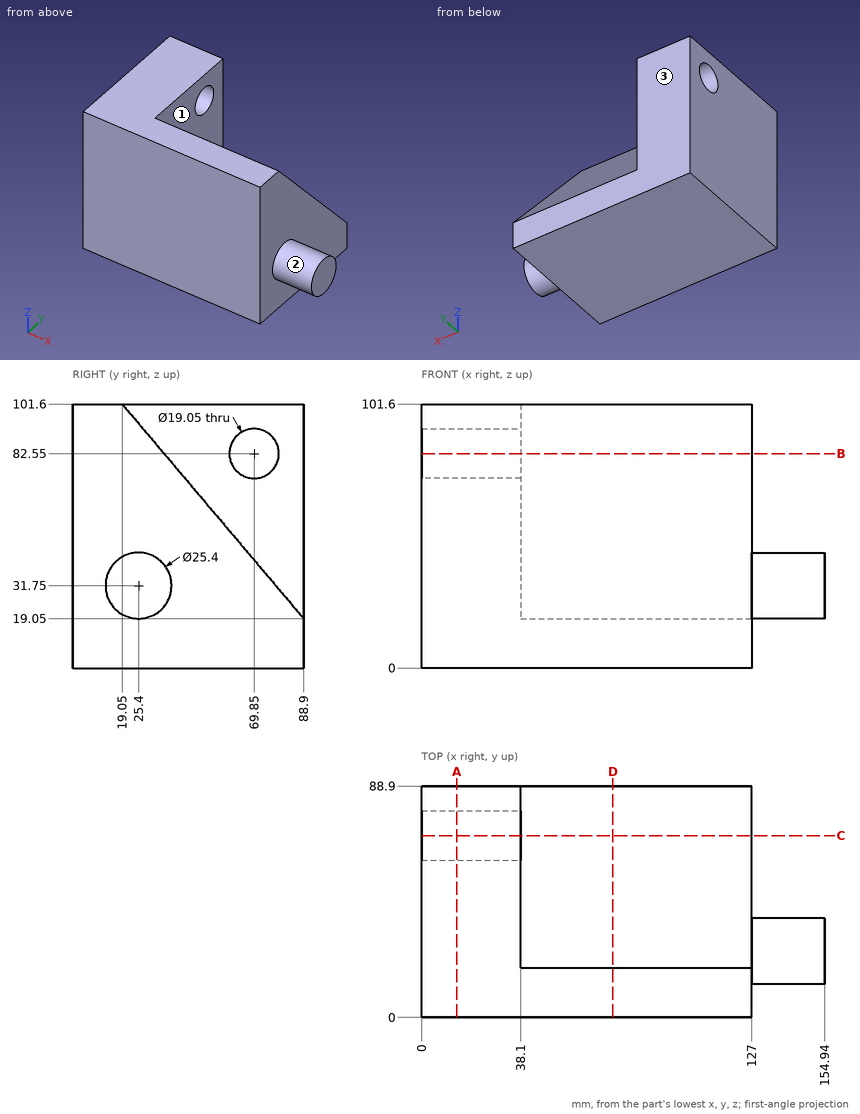
Answer from the drawing. Dimensions are ordinates in mm from the lowest x, y and z of the part. A direction names the side the tool comes from. Give positions to 0.01 mm unless a question says otherwise; leave off trailing zeros. Loops run counter-clockwise (first coordinate to the right, second up) from the corner with the lowest first, then second, coordinate; pieces in that order, holes last. Notation, with made-up numbers: M -28.5,61.25 L -1.5,61.25 A19 cw -1.5,73.25 Z; hole C -2.75,69 d6. An arc over 180 degrees is marked long. One line per item, written item: value.
Q1. A cutting plane is placed at D-D on x = 73.5. Determine the outline of the cut face in (y, z).
Working result:
outline: M 0,0 L 88.9,0 L 88.9,19.05 L 19.05,101.6 L 0,101.6 Z
Q2. Flat-ended cylindrical pins translate along their axes: P1, Ø1.5, axis at x = 108.5, y = 30.5, coming from the +Z side; P2, Ø21, axis at y = 56, z = 62, coming from the +X side; P3, Ø3, axis at x = 99, y = 75.5, coming from the +Z side; P4, Ø3, axis at y = 75, z = 88, coming from the -X side. Find the tip coordinate at first contact, or state that the pin passes through.
Working result:
P1: stops at z = 88.95
P2: stops at x = 127
P3: stops at z = 36.66
P4: passes through
Q3. A cutting plane is placed at C-C on y = 69.85. Determine the outline of the cut face in (x, z) (3 decimals), then the cut area to 3 significant figures.
Working result:
outline: M 0,0 L 127,0 L 127,41.564 L 38.1,41.564 L 38.1,73.025 L 0,73.025 Z; M 0,92.075 L 38.1,92.075 L 38.1,101.6 L 0,101.6 Z
area: 6,840 mm^2
Q4. A cutting plane is placed at A-A on x = 13.5. Determine the outline of the cut face in (y, z) (3 decimals), then the cut area to 3 significant figures.
Working result:
outline: M 0,0 L 88.9,0 L 88.9,101.6 L 0,101.6 Z; hole C 69.85,82.55 d19.05
area: 8,750 mm^2
Q5. Find the intervals of material crossed by line 1 (Z direction, x = 13, y = 69); line 2 (Y direction, x = 26.5, z = 82.55) (3 decimals); line 3 (X direction, y = 27.5, z = 6.5), in increasing order. Write a range as from..to.
Working result:
line 1: z = 0..73.06, 92.04..101.6
line 2: y = 0..60.325, 79.375..88.9
line 3: x = 0..127
Q6. For the marked faces 1, 2 and 3, determine the directions among +Z, -Z, +X, -X, +Y, -Y from which every point of the face is accessible in a straight line to the end or side of a thin tool.
Working result:
face 1: +Z, +X, +Y
face 2: +X
face 3: +Z, -Z, +X, -X, +Y
Q7. A cutting plane is placed at B-B on z = 82.55. Determine the outline of the cut face in (x, y) (3 decimals).
Working result:
outline: M 0,0 L 127,0 L 127,35.169 L 38.1,35.169 L 38.1,60.325 L 0,60.325 Z; M 0,79.375 L 38.1,79.375 L 38.1,88.9 L 0,88.9 Z
